Autodesk Inventor part; units mm, degrees
ref_plane "YZ Plane" through (0, 0, 0) normal (1, 0, 0) x (0, 1, 0)
ref_plane "XZ Plane" through (0, 0, 0) normal (0, 1, 0) x (-1, 0, 0)
ref_plane "XY Plane" through (0, 0, 0) normal (0, 0, 1) x (1, 0, 0)
sketch "Sketch1" plane through (0, 0, 0) normal (0, 1, 0) x (-1, 0, 0)
  line L0 (3.5, 3.5) -> (-3.5, 3.5)
  line L1 (-3.5, 3.5) -> (-3.5, -3.5)
  line L2 (-3.5, -3.5) -> (3.5, -3.5)
  line L3 (3.5, -3.5) -> (3.5, 3.5)
  line L4 (3.5, 2) -> (2, 3.5)
  line L5 (-2, -3.5) -> (-3.5, -2)
  point P0 (0, 0)
  dimension "d0" = 7
  dimension "d1" = 7
  dimension "d2" = 3.5
  dimension "d3" = 3.5
  dimension "d4" = 45
  dimension "d5" = 45
  dimension "d6" = 5.5
  dimension "d7" = 5.5
extrude "Extrusion1" add sketch "Sketch1" along normal blind 0.5 contours L4 L3 L2 L5 L1 L0
sketch "Sketch2" plane through (0, 0.5, 0) normal (0, 1, 0) x (1, 0, 0)
  circle A0 centre (0, 0) radius 3.5
  dimension "d10" = 7
extrude "Extrusion2" add sketch "Sketch2" along normal blind 4
sketch "Sketch3" plane through (0, 4.5, 0) normal (0, 1, 0) x (1, 0, 0)
  circle A0 centre (0, 0) radius 2.6934
  circle A1 centre (0, 0) radius 2.6335
extrude "Extrusion3" cut sketch "Sketch3" against normal blind 0.05
sketch "Sketch4" plane through (0, 0, 0) normal (0, -1, 0) x (1, 0, 0)
  line L0 (3.5, 3.5) -> (3.5, 0)
  line L1 (3.5, 1) -> (2, 1)
  line L2 (2, 1) -> (2, -1)
  line L3 (2, -1) -> (3.5, -1)
  line L4 (3.5, -1) -> (3.5, 1)
  line L5 (-2, 3.5) -> (3.5, 3.5)
  point P0 (0, 0)
  dimension "d15" = 1.5
  dimension "d16" = 2
  dimension "d17" = 2.5
extrude "Extrusion4" cut sketch "Sketch4" against normal blind 0.6
sketch "Sketch5" plane through (0, 0.6, 0) normal (0, -1, 0) x (1, 0, 0)
  line L0 (2, -1) -> (2, 1)
  line L1 (3.6, 1) -> (2, 1)
  line L2 (2, 1) -> (2, -1)
  line L3 (2, -1) -> (3.6, -1)
  line L4 (3.6, -1) -> (3.6, 1)
  point P0 (0, 0)
  dimension "d20" = 2
  dimension "d21" = 1.6
extrude "Extrusion5" add sketch "Sketch5" along normal blind 0.65
mirror "Mirror1" about plane through (0, 0, 0) normal (1, 0, 0) of "Extrusion4"
mirror "Mirror2" about plane through (0, 0, 0) normal (1, 0, 0) of "Extrusion5"
properties part number "SRR7045-151M"
Model file for the job. Use its own axes, mm. A direction names the side the tool comes from. Round coordinates to 2 decimals unless told otherwise and drop trailing zeros. Write each loop counter-clockwise with the first axis right and the second up, starting at its lowest first coordinate (ties: lowest second). Pieces come first, ordered by that corner, then holes. Notation, with made-up numbers: M 61.25,67.25 L 114.25,67.25 A11 cw 114.25,83.25 Z; hole C 47,19.25 d7. An arc over 180 degrees is marked long. Put each result on its own line as item: value.
Item 1: Cut at A-A (x = -2.5). List the corners of the cut face in (y, z), and give its area (3 significant figures).
Responses:
outline: M -0.05,-1 L 0,-1 L 0,-3.5 L 0.5,-3.5 L 0.5,-2.45 L 4.5,-2.45 L 4.5,-1 L 4.45,-1 L 4.45,-0.83 L 4.5,-0.83 L 4.5,0.83 L 4.45,0.83 L 4.45,1 L 4.5,1 L 4.5,2.45 L 0.5,2.45 L 0.5,3 L 0,3 L 0,1 L -0.05,1 Z
area: 22.9 mm²
Item 2: Cut at C-C (y = 1.5). List the corners of the cut face in (x, z), and give its area (3 significant figures).
Responses:
outline: C 0,0 d7
area: 38.5 mm²
Item 3: Probe L1, parallel to Y at x = 2.75, z = 2.25; L2, parallel to Y at x = 1.5, z = -1.25; L3, parallel to Z at x = 1, y = 1.7. List the from-to ranges inside material, lowest first. Write a range as from..to.
Responses:
L1: 0..0.5
L2: 0..4.5
L3: -3.35..3.35
Item 4: Cut at B-B (z = -3). List the corners of the cut face in (x, y).
Responses:
outline: M -3.5,0 L 2.5,0 L 2.5,0.5 L 1.8,0.5 L 1.8,4.5 L -1.8,4.5 L -1.8,0.5 L -3.5,0.5 Z
Item 5: Flat gauge pins, fed straight in: P1, Ø1, axis at x = -0.5, z = -0.5, coming from the -Y side; P2, Ø1.5, axis at x = 1, y = 1.5, coming from the -Z side; P3, Ø1, axis at y = 2, z = 0.5, coming from the +X side. Where does each tip first touch, or does it go through?
Responses:
P1: y = 0
P2: z = -3.49
P3: x = 3.5
Item 6: Tool access for faces 1 (the flat face through (3, 0.5, 3)), 2 (the flat face through (-3, 0.5, -3)), 3 (the flat face through (2.67, 0.5, -2.61)), 4 (the cylindrical face through (3.233, 2.472, -1.341)): list every direction of +Z, -Z, +X, -X, +Y, -Y with a clear straight run to the whole face (end or side of a thin tool).
Responses:
face 1: +Z, +X, +Y
face 2: -Z, -X, +Y
face 3: -Z, +X, +Y
face 4: +Y
Item 7: Cut at D-D (x = 1). List the corners of the cut face in (y, z), and give its area (3 significant figures).
Responses:
outline: M 0,-3.5 L 0.5,-3.5 L 0.5,-3.35 L 4.5,-3.35 L 4.5,-2.5 L 4.45,-2.5 L 4.45,-2.44 L 4.5,-2.44 L 4.5,2.44 L 4.45,2.44 L 4.45,2.5 L 4.5,2.5 L 4.5,3.35 L 0.5,3.35 L 0.5,3.5 L 0,3.5 Z
area: 30.3 mm²
